Here's how the part is built. I have some questions about the finished solid (model axes, mm). A direction names the side the tool comes from. Round coordinates to 2 decimals unless told otherwise and drop trailing zeros. Write each loop counter-clockwise with the first axis right and the second up, starting at its lowest first coordinate (ties: lowest second). Pieces come first, ordered by that corner, then holes. Notation, with made-up numbers: (24.25, 56.25) - (51.25, 56.25) arc R16 ccw to (51.25, 83.25) - close; hole circle Ø2 at (-9, -35.5). An arc over 180 degrees is marked (long way). Use one line per item in the form item = value. Start each with the question number.
1. If I drill on line 1 along Z through (x, y) = (-2.25, -7.25); line 2 along Y through (x, z) = (-2.5, 5); line 3 along Y through (x, z) = (0.5, 3.5), over which ranges is the centre line in solid material (lowest first)?
2. I want a section at C-C, the plane x = -1.75. List the corners of the cut face in (y, z) for me, plus the area to 3 significant figures.
3. I want a section at D-D, the plane y = -5. List the corners of the cut face in (x, z) for me.
4. I want a section at B-B, the plane z = 5.75. List the corners of the cut face in (x, y) for me.
5. I want a section at A-A, the plane y = -9. List the corners of the cut face in (x, z) for me.
6. Which directions (+Z, -Z, +X, -X, +Y, -Y) give clear straight access to the entire face, cutting with the end or side of a thin tool? Please do faces 1 (the flat face through (0, 0, 5)), 2 (the flat face through (0, -12, 5)), 3 (the cylindrical face through (-2.226, -8.943, 3.596)).
7. We'd pull the mould along Z, two halves only. Please class faces 4 (the flat face through (-2, 9, 5)), 5 (the cylindrical face through (-2.21, 2.662, 1.946)), 6 (the cylindrical face through (-3.05, -5.92, 9.05)): +Z half, -Z half, draft (parallel to the pull), parting line (faces both ways), or undercut.
8. Will this pin go through, and if not, where does the flat tip stop? pin 1 (0.8 mm diameter, centred on x = 2.5, y = -4.5, fed in from -Z).
Autodesk Inventor part; units mm, degrees
ref_plane "YZ Plane" through (0, 0, 0) normal (1, 0, 0) x (0, 1, 0)
ref_plane "XZ Plane" through (0, 0, 0) normal (0, 1, 0) x (-1, 0, 0)
ref_plane "XY Plane" through (0, 0, 0) normal (0, 0, 1) x (1, 0, 0)
sketch "Sketch1" plane through (0, 0, 0) normal (0, 1, 0) x (-1, 0, 0)
  circle A0 centre (2.1789, 5.1456) radius 4
  circle A1 centre (2.1789, 2.9456) radius 1
  circle A2 centre (2.1789, 5.1456) radius 1.75
  point P0 (0, 0)
  dimension "d0" = 8
  dimension "d1" = 2
  dimension "d3" = 3.5
  dimension "d4" = 0
  dimension "d5" = 0
  dimension "d6" = 0
  dimension "d17" = 2.2
extrude "Extrusion1" add sketch "Sketch1" against normal blind 3 contours A0 | A1 A2 | A2 A1 | A1 A2
extrude "Extrusion2" add sketch "Sketch1" along normal blind 5.4 contours A1 A2 | A2 A1 picked at (1.7556, 3.0976) picked at (2.385, 3.5861)
extrude "Extrusion3" add sketch "Sketch1" along normal blind 9 and the other way blind 12 contours A2 A1 | A1 A2 picked at (2.385, 3.5861) picked at (2.2193, 5.9034)
sketch "Sketch2" plane through (-2.1789, -12, 5.1456) normal (0, -1, 0) x (1, 0, 0)
  circle A0 centre (0, 0) radius 4
  circle A1 centre (0, 0) radius 1.55
  line L0 (-1.2619, 0.9) -> (1.2619, 0.9)
  circle A2 centre (0, 0) radius 4
  point P0 (2.1789, -5.1456)
  dimension "d18" = 8
  dimension "d19" = 3.1
  dimension "d20" = 2.45
extrude "Extrusion4" add sketch "Sketch2" against normal blind 9 contours A0 | A1 L0 | L0 A1
extrude "Extrusion5" cut sketch "Sketch2" against normal blind 6.2 contours A1 L0 picked at (-0.0386, 0.0848)
sketch "Sketch3" plane through (-2.1789, 0, 5.1456) normal (0, 1, 0) x (1, 0, 0)
  line L0 (3.7119, 0.25) -> (4.7119, 0.25)
  line L1 (4.7119, 0.25) -> (4.7119, -0.25)
  line L2 (4.7119, -0.25) -> (3.7119, -0.25)
  line L3 (3.7119, -0.25) -> (3.7119, 0.25)
  circle A0 centre (0, 0) radius 4
  point P0 (2.1789, 5.1456)
  dimension "d25" = 0.5
  dimension "d26" = 0.25
  dimension "d27" = 0.25
  dimension "d30" = 1
extrude "Extrusion6" add sketch "Sketch3" against normal blind 10 contours L0 A0 L2 L3 | L0 L1 L2 A0 picked at (3.8079, 0)
sketch "Sketch4" plane through (0, 0, 0) normal (0, 1, 0) x (1, 0, 0)
  line L0 (1.8133, -4.8956) -> (2.5329, -4.8956)
  line L1 (2.5329, -5.3956) -> (1.8133, -5.3956)
  line L2 (2.5329, -4.8956) -> (1.8133, -4.8956)
  line L3 (1.8133, -4.8956) -> (1.8133, -5.3956)
  line L4 (1.8133, -5.3956) -> (2.5329, -5.3956)
  line L5 (2.5329, -5.3956) -> (2.5329, -4.8956)
  point P0 (0, 0)
extrude "Extrusion7" cut sketch "Sketch4" against normal blind 2
properties part number "kolo"
Model answer:
q1.line_1 = 1.15 to 3.6, 6.05 to 9.14
q1.line_2 = -5.8 to 9
q1.line_3 = -12 to 0
q2.outline = (-12, 1.17) - (0, 1.17) - (0, 2.04) - (5.4, 2.04) - (5.4, 3.45) - (9, 3.45) - (9, 6.84) - (0, 6.84) - (0, 9.12) - (-12, 9.12) - (-12, 6.05) - (-5.8, 6.05) - (-5.8, 3.66) - (-12, 3.66) - close
q2.area = 119 mm2
q3.outline = (1.81, 4.9) - (2.53, 4.9) - (2.53, 5.4) - (1.81, 5.4) arc R4 ccw (long way) to start
q4.outline = (-6.13, -12) - (-3.61, -12) - (-3.61, -5.8) - (-0.75, -5.8) - (-0.75, -12) - (1.78, -12) - (1.78, 0) - (-0.54, 0) - (-0.54, 9) - (-3.82, 9) - (-3.82, 0) - (-6.13, 0) - close
q5.outline = (1.81, 4.9) - (2.53, 4.9) - (2.53, 5.4) - (1.81, 5.4) arc R4 ccw (long way) to start; hole (-3.44, 6.05) arc R1.55 ccw (long way) to (-0.92, 6.05) - close
q6.face_1 = +Y
q6.face_2 = +Z, -Z, +X, -X, -Y
q6.face_3 = -Y
q7.face_4 = draft
q7.face_5 = undercut
q7.face_6 = parting line
q8.pin_1 = 4.9
